Geometry: see drawing. Coordinates: mm, zero at the bounding-box minimum. Coordinates: 2 decimals unless noted, no trailing zeros. Loops run counter-clockwise (first coordinate to the right, second up) from the corner with the lowest first, then second, coordinate; pieces in that order, holes last. Notation, with made-up numbers: (53, -19) - (110, -19) arc R18 ccw to (110, 13) - close; hole circle Ø9 at (8, -16). An arc over 180 degrees is marked (long way). Use a Markdown table: item, result. Add a question column.
1. Ray query, L1, parallel to X at y = 5.3, z = 20; L2, parallel to Y at x = 107, z = 14; L3, parallel to Z at x = 40, y = 2.85. Return the intervals inside material, ascending. Write a range as [from, to].
2. Section query A-A on z = 20. Return the cut outline in (x, y).
3. Section query B-B on y = 2.85. Return the cut outline in (x, z) (1 decimal), then the cut area to 3 significant figures.
4. Section query C-C on x = 125. Return the cut outline in (y, z).
5. Draft query along X for the marked faces 1 and 2. Return one class per face: released by +X, released by -X, zero draft, split by the parting line, or undercut.
6. Contact query for flat-ended pins moving along their axis: P1, Ø2.5, axis at x = 15, z = 20, coming from the -Y side; P2, Ø5, axis at x = 125, z = 20, coming from the -Y side; P3, Ø1, axis at y = 2, z = 28.5, coming from the -X side; P4, Ø3, axis at x = 53.5, y = 1, coming from the -Z side. Output: stop coordinate, or through.
7. Section query D-D on x = 15. Return the cut outline in (y, z).
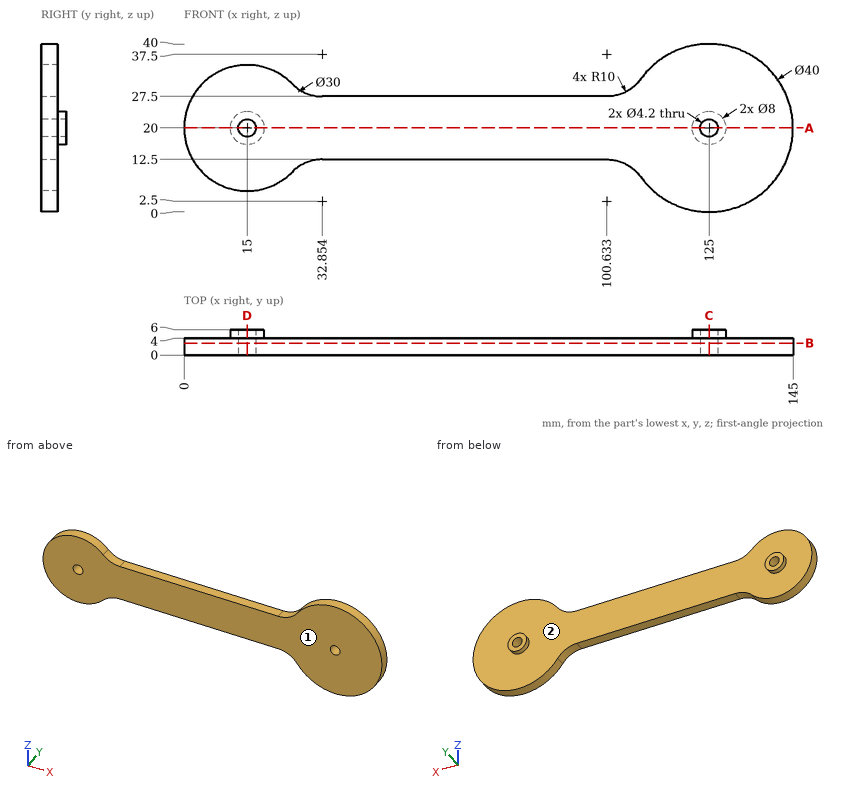
Resolved:
| question | item | result |
|---|---|---|
| 1 | L1 | [11, 12.9], [17.1, 19], [121, 122.9], [127.1, 129] |
| 1 | L2 | [0, 4] |
| 1 | L3 | [12.5, 27.5] |
| 2 | outline | (0, 0) - (12.9, 0) - (12.9, 6) - (11, 6) - (11, 4) - (0, 4) - close; (17.1, 0) - (122.9, 0) - (122.9, 6) - (121, 6) - (121, 4) - (19, 4) - (19, 6) - (17.1, 6) - close; (127.1, 0) - (145, 0) - (145, 4) - (129, 4) - (129, 6) - (127.1, 6) - close |
| 3 | outline | (25.7, 9.5) arc R10 cw to (32.9, 12.5) - (100.6, 12.5) arc R10 cw to (108.8, 8.3) arc R20 ccw (long way) to (108.8, 31.7) arc R10 cw to (100.6, 27.5) - (32.9, 27.5) arc R10 cw to (25.7, 30.5) arc R15 ccw (long way) to start; hole circle Ø4.2 at (15, 20); hole circle Ø4.2 at (125, 20) |
| 3 | area | 3,090 mm² |
| 4 | outline | (0, 0) - (4, 0) - (4, 16) - (6, 16) - (6, 17.9) - (0, 17.9) - close; (0, 22.1) - (6, 22.1) - (6, 24) - (4, 24) - (4, 40) - (0, 40) - close |
| 5 | face 1 | zero draft |
| 5 | face 2 | undercut |
| 6 | P1 | through |
| 6 | P2 | y = 0 |
| 6 | P3 | x = 2.31 |
| 6 | P4 | z = 12.5 |
| 7 | outline | (0, 5) - (4, 5) - (4, 16) - (6, 16) - (6, 17.9) - (0, 17.9) - close; (0, 22.1) - (6, 22.1) - (6, 24) - (4, 24) - (4, 35) - (0, 35) - close |
